Autodesk Inventor part; units mm, degrees
ref_plane "YZ Plane" through (0, 0, 0) normal (1, 0, 0) x (0, 1, 0)
ref_plane "XZ Plane" through (0, 0, 0) normal (0, 1, 0) x (-1, 0, 0)
ref_plane "XY Plane" through (0, 0, 0) normal (0, 0, 1) x (1, 0, 0)
sketch "스케치1" plane through (0, 0, 0) normal (0, 0, 1) x (1, 0, 0)
  circle A0 centre (0, 0) radius 2.5
  line L0 (-6.35, 0) -> (6.35, 0) construction
  line L1 (-6.35, -1.9) -> (6.35, -1.9)
  line L2 (6.35, 1.9) -> (-6.35, 1.9)
  arc A1 (-6.35, 1.9) -> (-6.35, -1.9) centre (-6.35, 0) ccw
  arc A2 (6.35, -1.9) -> (6.35, 1.9) centre (6.35, 0) ccw
  line L3 (0, 14.5) -> (0, -14.5) construction
  circle A3 centre (0, 14.5) radius 0.5
  circle A4 centre (0, -14.5) radius 0.5
  circle A5 centre (6.35, 0) radius 0.5
  circle A6 centre (-6.35, 0) radius 0.5
  circle A7 centre (-4.25, 0) radius 0.5
  circle A8 centre (4.25, 0) radius 0.5
  line L4 (0, -1.9) -> (0, -18.5)
  line L5 (0, 1.9) -> (0, 15.9)
  arc A9 (1.9954, 14.0355) -> (-1.9954, 14.0355) centre (0, 13.9) ccw
  arc A10 (-1.9969, -16.6117) -> (1.9969, -16.6117) centre (0, -16.5) ccw
  circle A11 centre (0, 0) radius 3.4
  line L6 (-1.9954, 14.0355) -> (-2.8196, 1.9)
  line L7 (1.9954, 14.0355) -> (2.8196, 1.9)
  line L8 (-2.8196, -1.9) -> (-1.9969, -16.6117)
  line L9 (2.8196, -1.9) -> (1.9969, -16.6117)
  circle A12 centre (0, 12.5) radius 0.5
  circle A13 centre (0, 10.5) radius 0.5
  circle A14 centre (0, 8.5) radius 0.5
  circle A15 centre (0, 6.5) radius 0.5
  circle A16 centre (0, 4.5) radius 0.5
  circle A17 centre (0, 0) radius 2.35
  circle A18 centre (0, -16.5) radius 0.5
  circle A19 centre (0, -12.5) radius 0.5
  circle A20 centre (0, -10.5) radius 0.5
  circle A21 centre (0, -8.5) radius 0.5
  circle A22 centre (0, -6.5) radius 0.5
  circle A23 centre (0, -4.5) radius 0.5
  dimension "d0" = 5
  dimension "d1" = 1.9
  dimension "d2" = 16.5
  dimension "d3" = 29
  dimension "d4" = 1
  dimension "d5" = 1
  dimension "d6" = 1
  dimension "d7" = 1
  dimension "d10" = 2.1
  dimension "d17" = 2.1
  dimension "d24" = 16.6
  dimension "d25" = 14
  dimension "d26" = 4
  dimension "d27" = 4
  dimension "d28" = 6.8
  dimension "d31" = 2
  dimension "d36" = 4.7
  dimension "d39" = 2
  dimension "d46" = 2
extrude "돌출1" add sketch "스케치1" along normal blind 2.2 contours A0 L1 A17 L2 | A0 L2 A11 L1 | L2 A17 L5 A0 | A0 L5 A11 L2 | L1 A11 L4 A0 | A0 L4 A17 L1 | L5 A17 L2 A0 | A0 L2 A11 L5 | A17 L1 L2 | L2 L5 A17 | L4 A11 L1 A0 | A0 L1 A17 L4 | A17 L4 L1 | L2 A17 L1 A0 | A0 L1 A11 L2 | L5 L2 A17 | A17 L1 L4
extrude "돌출2" add sketch "스케치1" against normal blind 2.11 contours A0 L1 A17 L2 | A0 L2 A11 L1 | L2 A17 L5 A0 | A0 L5 A11 L2 | L1 A11 L4 A0 | A0 L4 A17 L1 | L5 A17 L2 A0 | A0 L2 A11 L5 | L2 A2 L1 A11 | A11 L5 A16 A15 A14 A13 A12 A3 A9 L7 | A17 L1 L2 | L2 L5 A17 | L4 A11 L1 A0 | A0 L1 A17 L4 | A17 L4 L1 | L9 A10 L4 A18 A4 A19 A20 A21 A22 A23 A11 | L2 A17 L1 A0 | A0 L1 A11 L2 | L5 L2 A17 | A11 L6 A9 L5 A3 A12 A13 A14 A15 A16 | A17 L1 L4 | L4 A23 A22 A21 A20 A19 A4 A18 A10 L8 A11 | A11 L1 A1 L2
extrude "돌출3" cut sketch "스케치1" along normal blind 3.65 contours A17 L1 L2 | L2 L5 A17 | A17 L4 L1 | L5 L2 A17 | A17 L1 L4
sketch "스케치2" plane through (0, 0, 0) normal (0, 0, 1) x (1, 0, 0)
  circle A0 centre (0, 0) radius 1.25
  dimension "d57" = 2.5
extrude "돌출4" cut sketch "스케치2" against normal blind 7.6
sketch "스케치3" plane through (0, 0, -2.11) normal (0, 0, -1) x (-1, 0, 0)
  circle A0 centre (0, 0) radius 2.25
  dimension "d60" = 4.5
extrude "돌출5" cut sketch "스케치3" against normal blind 1
sketch "스케치4" plane through (0, 0, -2.11) normal (0, 0, -1) x (-1, 0, 0)
  point P0 (0, 0)
sketch "스케치5" plane through (0, 0, -2.11) normal (0, 0, -1) x (-1, 0, 0)
  circle A0 centre (0, 0) radius 3.4
  circle A1 centre (0, 0) radius 2.25
  dimension "d63" = 4.5
  dimension "d64" = 6.8
extrude "돌출6" add sketch "스케치5" along normal blind 0.4
sketch "스케치6" plane through (0, 0, -2.11) normal (0, 0, -1) x (-1, 0, 0)
  line L0 (0.9014, 15.3127) -> (-1.0592, 15.3127)
  line L1 (-1.0592, 15.3127) -> (-1.0592, 3.6394)
  line L2 (-1.0592, 3.6394) -> (0.9014, 3.6394)
  line L3 (0.9014, 3.6394) -> (0.9014, 15.3127)
  line L4 (1.0141, -3.7747) -> (-1.0592, -3.7747)
  line L5 (-1.0592, -3.7747) -> (-1.0592, -17.386)
  line L6 (-1.0592, -17.386) -> (1.0141, -17.386)
  line L7 (1.0141, -17.386) -> (1.0141, -3.7747)
  point P0 (0, 0)
extrude "돌출7" add sketch "스케치6" against normal blind 2.11
sketch "스케치7" plane through (0, 0, -2.11) normal (0, 0, -1) x (-1, 0, 0)
  circle A0 centre (0, 14.3) radius 0.5
  arc A1 (1.9954, 14.0355) -> (-1.9954, 14.0355) centre (0, 13.9) ccw
  line L0 (0, 0) -> (0, 0.7105)
  line L1 (0, 0) -> (0.8275, 0)
  circle A2 centre (0, 12.3) radius 0.5
  circle A3 centre (0, 10.3) radius 0.5
  circle A4 centre (0, 8.3) radius 0.5
  circle A5 centre (0, 6.3) radius 0.5
  circle A6 centre (0, 4.3) radius 0.5
  line L2 (0, 15.9) -> (3.4178, 15.9)
  arc A7 (1.9954, 14.0355) -> (-1.9954, 14.0355) centre (0, 13.9) ccw
  circle A8 centre (0, -16.9) radius 0.5
  arc A9 (-1.9969, -16.6117) -> (1.9969, -16.6117) centre (0, -16.5) ccw
  circle A10 centre (0, -14.9) radius 0.5
  circle A11 centre (0, -12.9) radius 0.5
  circle A12 centre (0, -10.9) radius 0.5
  circle A13 centre (0, -8.9) radius 0.5
  circle A14 centre (0, -6.9) radius 0.5
  circle A15 centre (0, -4.9) radius 0.5
  point P0 (0, -18.5)
  dimension "d69" = 1
  dimension "d73" = 2
  dimension "d78" = 1.6
  dimension "d79" = 1
  dimension "d80" = 1.6
  dimension "d86" = 2
extrude "돌출8" cut sketch "스케치7" against normal blind 2.11
sketch "스케치9" plane through (0, 0, -2.11) normal (0, 0, -1) x (-1, 0, 0)
  circle A0 centre (0, 8.3) radius 0.5
  line L0 (0.5, 8.3) -> (3.8465, 8.3)
  line L1 (3.8465, 8.3) -> (3.8465, 17.7965)
  line L2 (3.8465, 17.7965) -> (-4.3088, 17.7965)
  line L3 (-4.3088, 17.7965) -> (-4.3088, 8.3)
  line L4 (-4.3088, 8.3) -> (0.2806, 8.3)
  circle A1 centre (0, -8.9) radius 0.5
  line L5 (0, -8.9) -> (5.2333, -8.9)
  line L6 (5.2333, -8.9) -> (5.2333, -19.7775)
  line L7 (5.2333, -19.7775) -> (-4.9031, -19.7775)
  line L8 (-4.9031, -19.7775) -> (-4.9031, -8.9)
  line L9 (-4.9031, -8.9) -> (0, -8.9)
  point P0 (0, 0)
  point P1 (0.5, -8.9)
  point P2 (-0.5, -8.9)
  point P3 (-0.5, 8.3)
extrude "돌출9" cut sketch "스케치9" against normal blind 10 contours A0 L4 L3 L2 L1 L0 | L5 L6 L7 L8 L9 A1
sketch "스케치10" plane through (0, 0, -2.11) normal (0, 0, -1) x (-1, 0, 0)
  line L0 (-0.0004, 7.8) -> (4.3151, 7.8)
  line L1 (4.3151, 7.8) -> (3.7805, 10.6296)
  line L2 (3.7805, 10.6296) -> (-3.3513, 10.6296)
  line L3 (-3.3513, 10.6296) -> (-3.4414, 7.8)
  line L4 (-3.4414, 7.8) -> (-0.0004, 7.8)
  arc A0 (-0.5, 8.3) -> (0.5, 8.3) centre (0, 8.3) ccw
  arc A1 (0.5, -8.9) -> (-0.5, -8.9) centre (0, -8.9) ccw
  line L5 (0, -8.4) -> (4.5069, -8.4)
  line L6 (4.5069, -8.4) -> (4.5069, -10.1694)
  line L7 (4.5069, -10.1694) -> (-4.0138, -10.1694)
  line L8 (-4.0138, -10.1694) -> (-4.0138, -8.4)
  line L9 (-4.0138, -8.4) -> (0, -8.4)
  point P0 (0, 0)
extrude "돌출10" cut sketch "스케치10" against normal blind 10
fillet "모깎기1" radius 2 4 edges at (2.4189, 7.8, -1.055) (-2.4189, 7.8, -1.055) (-2.4561, -8.4, -1.055) (2.4561, -8.4, -1.055)
sketch "스케치11" plane through (0, 0, -2.11) normal (0, 0, -1) x (-1, 0, 0)
  line L0 (-6.35, -1.9) -> (-2.8196, -1.9)
  line L1 (-2.8196, 1.9) -> (-6.35, 1.9)
  circle A0 centre (0, 6.3) radius 0.5
  circle A1 centre (0, -6.9) radius 0.5
  line L2 (2.8196, 1.9) -> (2.5455, 5.9355)
  line L3 (-2.5455, 5.9355) -> (-2.8196, 1.9)
  line L4 (0.5501, 7.8) -> (-0.5501, 7.8)
  line L5 (-2.8196, -1.9) -> (-2.5617, -6.5117)
  line L6 (2.5617, -6.5117) -> (2.8196, -1.9)
  point P0 (0, 0)
  point P1 (-4.5848, -1.9)
  point P2 (-4.5848, 1.9)
  point P3 (0, 7.8)
  dimension "d95" = 3.8
  dimension "d96" = 6.3
  dimension "d97" = 6.9
  dimension "d98" = 7.77
  dimension "d99" = 7.8
  dimension "d100" = 6.401
sketch "스케치12" plane through (0, 0, -2.11) normal (0, 0, -1) x (-1, 0, 0)
  line L0 (2.5785, 5.3) -> (-2.5887, 5.3)
  line L1 (-2.5455, 5.9355) -> (-2.8196, 1.9)
  circle A0 centre (0, 4.3) radius 0.5
  line L2 (3.3006, -5.9) -> (-2.5959, -5.9)
  line L3 (-2.8196, -1.9) -> (-2.5617, -6.5117)
  circle A1 centre (0, -4.9) radius 0.5
  line L4 (2.8196, 1.9) -> (6.35, 1.9)
  line L5 (5.3, 1.9) -> (5.3, -1.9)
  circle A2 centre (4.25, 0) radius 0.5
  line L6 (-6.35, 1.9) -> (-2.8196, 1.9)
  line L7 (-5.3, 1.9) -> (-5.3, -2.6397)
  circle A3 centre (-4.25, 0) radius 0.5
  line L8 (5.3, 1.9) -> (9.4862, 1.9)
  line L9 (9.4862, 1.9) -> (9.4862, -2.8158)
  line L10 (9.4862, -2.8158) -> (5.3, -2.8158)
  line L11 (5.3, -2.8158) -> (5.3, 1.9)
  line L12 (3.3006, -5.9) -> (-3.636, -5.9)
  line L13 (-3.636, -5.9) -> (-3.636, -9.5734)
  line L14 (-3.636, -9.5734) -> (3.3006, -9.5734)
  line L15 (3.3006, -9.5734) -> (3.3006, -5.9)
  line L16 (-5.3, -2.6397) -> (-8.4677, -2.6397)
  line L17 (-8.4677, -2.6397) -> (-8.4677, 1.9)
  line L18 (-8.4677, 1.9) -> (-5.3, 1.9)
  line L19 (-5.3, 1.9) -> (-5.3, -2.6397)
  line L20 (-2.5887, 5.3) -> (3.3006, 5.3)
  line L21 (3.3006, 5.3) -> (3.3006, 8.0343)
  line L22 (3.3006, 8.0343) -> (-2.5887, 8.0343)
  line L23 (-2.5887, 8.0343) -> (-2.5887, 5.3)
  point P0 (0, 0)
  point P1 (-0.0051, 5.3)
  point P2 (-2.5617, -5.9)
  point P3 (-2.5959, -5.9)
  dimension "d101" = 1
  dimension "d102" = 1
  dimension "d104" = 1.05
  dimension "d105" = 1.05
extrude "돌출11" cut sketch "스케치12" against normal blind 10 contours L0 L23 L22 L21 L20 | L15 L14 L13 L12 L2 | L4 L8 L9 L10 L11 L5 | L6 L7 L16 L17 L18
sketch "스케치14" plane through (0, 0, -2.11) normal (0, 0, -1) x (-1, 0, 0)
  line L0 (2.5887, 5.3) -> (-2.5887, 5.3)
  line L1 (-2.5887, 5.3) -> (-2.8196, 1.9)
  arc A0 (2.8196, 1.9) -> (-2.8196, 1.9) centre (0, 0) ccw
  line L2 (2.8196, 1.9) -> (2.5887, 5.3)
  circle A1 centre (0, 4.3) radius 0.5
  circle A2 centre (0, 0) radius 3.4
  circle A3 centre (0, 0) radius 2.25
  line L3 (5.3, -1.9) -> (5.3, 1.9)
  line L4 (5.3, 1.9) -> (2.8196, 1.9)
  arc A4 (2.8196, -1.9) -> (2.8196, 1.9) centre (0, 0) ccw
  line L5 (2.8196, -1.9) -> (5.3, -1.9)
  circle A5 centre (4.25, 0) radius 0.5
  line L6 (-2.5959, -5.9) -> (2.5959, -5.9)
  line L7 (2.5959, -5.9) -> (2.8196, -1.9)
  arc A6 (-2.8196, -1.9) -> (2.8196, -1.9) centre (0, 0) ccw
  line L8 (-2.8196, -1.9) -> (-2.5959, -5.9)
  circle A7 centre (0, -4.9) radius 0.5
  line L9 (-5.3, 1.9) -> (-5.3, -1.9)
  line L10 (-5.3, -1.9) -> (-2.8196, -1.9)
  arc A8 (-2.8196, 1.9) -> (-2.8196, -1.9) centre (0, 0) ccw
  line L11 (-2.8196, 1.9) -> (-5.3, 1.9)
  circle A9 centre (-4.25, 0) radius 0.5
  circle A10 centre (0, 0) radius 1.25
  circle A11 centre (0, 0) radius 2.25
  circle A12 centre (0, 0) radius 7.35
  point P0 (2.8196, -1.9)
  dimension "d111" = 14.7
sketch "스케치15" plane through (0, 0, -2.51) normal (0, 0, -1) x (-1, 0, 0)
  line L0 (-8.2432, 8.5445) -> (15.2986, 8.5445)
  line L1 (15.2986, 8.5445) -> (15.2986, -14.1463)
  line L2 (15.2986, -14.1463) -> (-8.2432, -14.1463)
  line L3 (-8.2432, -14.1463) -> (-8.2432, 8.5445)
  point P0 (0, 0)
extrude "돌출12" cut sketch "스케치15" along normal mid plane 10
extrude "돌출13" add sketch "스케치14" along normal blind 3 contours A12
sketch "스케치16" plane through (0, 0, -5.11) normal (0, 0, -1) x (-1, 0, 0)
  circle A0 centre (0, 0) radius 4
  circle A1 centre (0, 0) radius 7.35
  circle A2 centre (0, 0) radius 7.35
  dimension "d114" = 8
extrude "돌출14" add sketch "스케치16" along normal blind 0.5
sketch "스케치17" plane through (0, 0, -2.11) normal (0, 0, 1) x (1, 0, 0)
  circle A0 centre (0, 0) radius 7.35
  line L0 (2.5887, 5.3) -> (-2.5887, 5.3)
  line L1 (2.8196, 1.9) -> (2.5887, 5.3)
  line L2 (5.3, 1.9) -> (2.8196, 1.9)
  line L3 (5.3, -1.9) -> (5.3, 1.9)
  line L4 (2.8196, -1.9) -> (5.3, -1.9)
  line L5 (2.5959, -5.9) -> (2.8196, -1.9)
  line L6 (-2.5959, -5.9) -> (2.5959, -5.9)
  line L7 (-2.8196, -1.9) -> (-2.5959, -5.9)
  line L8 (-5.3, -1.9) -> (-2.8196, -1.9)
  line L9 (-5.3, 1.9) -> (-5.3, -1.9)
  line L10 (-2.8196, 1.9) -> (-5.3, 1.9)
  line L11 (-2.5887, 5.3) -> (-2.8196, 1.9)
  line L12 (-2.7755, 5.5) -> (2.7755, 5.5)
  line L13 (2.7755, 5.5) -> (3.0065, 2.1)
  line L14 (3.0065, 2.1) -> (5.5, 2.1)
  line L15 (5.5, 2.1) -> (5.5, -2.1)
  line L16 (5.5, -2.1) -> (3.0087, -2.1)
  line L17 (3.0087, -2.1) -> (2.785, -6.1)
  line L18 (2.785, -6.1) -> (-2.785, -6.1)
  line L19 (-2.785, -6.1) -> (-3.0087, -2.1)
  line L20 (-3.0087, -2.1) -> (-5.5, -2.1)
  line L21 (-5.5, -2.1) -> (-5.5, 2.1)
  line L22 (-5.5, 2.1) -> (-3.0065, 2.1)
  line L23 (-3.0065, 2.1) -> (-2.7755, 5.5)
  dimension "d117" = 0.2
extrude "돌출15" cut sketch "스케치17" against normal blind 3 contours L1 L2 L3 L4 L5 L6 L7 L8 L9 L10 L11 L0 | L12 L13 L14 L15 L16 L17 L18 L19 L20 L21 L22 L23
fillet "모깎기2" radius 1 4 edges at (-3.0065, 2.1, -3.61) (3.0065, 2.1, -3.61) (3.0087, -2.1, -3.61) (-3.0087, -2.1, -3.61)
sketch "스케치18" plane through (0, 0, -5.61) normal (0, 0, -1) x (-1, 0, 0)
  circle A0 centre (0, 0) radius 12
  dimension "d121" = 24
extrude "돌출16" add sketch "스케치18" along normal blind 1.9
sketch "스케치19" plane through (0, 0, -7.51) normal (0, 0, -1) x (-1, 0, 0)
  circle A0 centre (0, 0) radius 24.5
  circle A1 centre (0, 18) radius 1.25
  circle A2 centre (-18, 0) radius 1.25
  circle A3 centre (0, -18) radius 1.25
  circle A4 centre (18, 0) radius 1.25
  dimension "d124" = 49
  dimension "d125" = 2.5
  dimension "d126" = 18
  dimension "d129" = 360
extrude "돌출17" add sketch "스케치19" along normal blind 3
sketch "스케치20" plane through (0, 0, -5.61) normal (0, 0, 1) x (1, 0, 0)
  circle A0 centre (0, 0) radius 4
  circle A1 centre (0, 0) radius 3
  dimension "d133" = 6
extrude "돌출18" cut sketch "스케치20" against normal blind 16 contours A1
properties part number "180도 서보모터 십자축"
CAD build for the part. Positions are in the model's coordinates, mm. A direction names the side the tool comes from. Coordinates: 2 decimals unless noted, no trailing zeros. Loops run counter-clockwise (first coordinate to the right, second up) from the corner with the lowest first, then second, coordinate; pieces in that order, holes last. Notation, with made-up numbers: (16, 10) - (26, 10) arc R16 cw to (26, 32) - close; hole circle Ø5 at (43, 16). An arc over 180 degrees is marked (long way). Return JSON: item names as keys, results as strings.
1. Band-saw the part on C-C (x = -18). Give the cut face in (y, z), and give its area (3 significant figures).
Result:
{"outline": "(-16.62, -10.51) - (-1.25, -10.51) - (-1.25, -7.51) - (-16.62, -7.51) - close; (1.25, -10.51) - (16.62, -10.51) - (16.62, -7.51) - (1.25, -7.51) - close", "area": "92.2 mm2"}
2. Drop flat-ended pins along their axis: pin 1 (4 mm diameter, centred on x = 19, z = -8.5, fed in from -Y); pin 2 (0.8 mm diameter, centred on x = 4.5, z = -3, fed in from +Y); pin 3 (1.7 mm diameter, centred on x = 4.5, z = -3.5, fed in from -Y). Give the stop position or say it passes through.
Result:
{"pin 1": "stops at y = -17.64", "pin 2": "stops at y = 6.1", "pin 3": "stops at y = -6.38"}
3. Mould opens along X. For faces 3 (the flat face through (2.87, -4.55, -3.59)), 4 (the flat face through (0, -6.1, -4)), 5 (the cylindrical face through (-13.17, -20.66, -8.99)), 6 (the flat face through (-5, 0, -10.51)) say: released by +X, released by -X, zero draft, split by the parting line, or undercut.
Result:
{"face 3": "undercut", "face 4": "undercut", "face 5": "split by the parting line", "face 6": "zero draft"}
4. Probe L1, parallel to Y at x = 0, z = -5.35; L2, parallel to Y at x = 0, z = -7.95; L3, parallel to Z at x = -20.5, y = 9. List the from-to ranges inside material, lowest first. Write a range as from..to.
Result:
{"L1": "y = -7.35..-4, 4..7.35", "L2": "y = -24.5..-19.25, -16.75..-3, 3..16.75, 19.25..24.5", "L3": "z = -10.51..-7.51"}
5. 3-axis set-ups, long thin cutter, end or side, ignore diameter. For faces 1 (the flat face through (2.86, 4.28, -3.59)), 2 (the cylindrical face through (0.27, -16.78, -8.99)): which of +Z, -Z, +X, -X, +Y, -Y reach the whole face in a straight line?
Result:
{"face 1": "+Z", "face 2": "+Z, -Z"}
6. Band-saw the part on A-A (y = 0). State how many separate pieces and enclosed holes the cut face has, and give its area (3 significant figures).
Result:
{"separate pieces": "4", "enclosed holes": "0", "area": "163 mm2"}
